Read the model definition and answer for the solid it produces. Units are mm, in the model's axes. A direction names the side the tool comes from. Give positions to 0.01 mm unless a question says otherwise; leave off trailing zeros. Write each loop counter-clockwise with the first axis right and the second up, starting at its lowest first coordinate (ties: lowest second). Pieces come first, ordered by that corner, then holes. Notation, with made-up numbers: (59.5, -30) - (89.5, -30) arc R25 ccw to (89.5, -15) - close; hole circle Ø6 at (36.5, -29). An arc over 180 degrees is marked (long way). Answer as a JSON object with one key per item and string values. Group by question number.
```python
from build123d import *

# Parameters (mm, degrees)
SKETCH1_W           = 40
SKETCH1_H           = 40
SKETCH1_R           = 2
SKETCH1_R_2         = 1.2
BOSS_EXTRUDE1_DEPTH = 4
SKETCH2_W           = 40
SKETCH2_H           = 40
BOSS_EXTRUDE2_DEPTH = 4
SKETCH3_W           = 7.5
SKETCH3_H           = 4
SKETCH3_W_2         = 20
SKETCH3_H_2         = 8
CUT_EXTRUDE1_DEPTH  = 4


with BuildPart() as part:
    # Sketch1 → Boss-Extrude1 (new body)
    with BuildSketch(Plane(origin=(0, 0, 0), x_dir=(1, 0, 0), z_dir=(0, 1, 0))):
        Rectangle(SKETCH1_W, SKETCH1_H)
        with Locations(Location((0, 0, 0), (0, 0, 270))):
            Circle(SKETCH1_R, mode=Mode.SUBTRACT)
        with Locations(Location((7, 0, 0), (0, 0, 270))):
            Circle(SKETCH1_R_2, mode=Mode.SUBTRACT)
        with Locations(Location((0, -7, 0), (0, 0, 270))):
            Circle(SKETCH1_R_2, mode=Mode.SUBTRACT)
        with Locations(Location((-7, 0, 0), (0, 0, 270))):
            Circle(SKETCH1_R_2, mode=Mode.SUBTRACT)
        with Locations(Location((0, 7, 0), (0, 0, 270))):
            Circle(SKETCH1_R_2, mode=Mode.SUBTRACT)
    extrude(amount=BOSS_EXTRUDE1_DEPTH)

    # Sketch2 → Boss-Extrude2 (add)
    with BuildSketch(Plane.XY.offset(20)):
        with Locations((0, 20)):
            Rectangle(SKETCH2_W, SKETCH2_H)
    extrude(amount=-BOSS_EXTRUDE2_DEPTH)

    # Sketch3 → Cut-Extrude1 (cut)
    with BuildSketch(Plane.XY.offset(20)):
        with Locations((-9.75, 30)):
            Rectangle(SKETCH3_W, SKETCH3_H)
        with Locations((9.75, 30)):
            Rectangle(SKETCH3_W, SKETCH3_H)
        with Locations((0, 12)):
            Rectangle(SKETCH3_W_2, SKETCH3_H_2)
    extrude(amount=-CUT_EXTRUDE1_DEPTH, mode=Mode.SUBTRACT)


solid = part.part
```
1) Find section D-D, the plane z = 7. Write down the section's boundary in (x, y), and give its area (3 significant figures).
2) Find the intervals of material crossed by line 1 (X direction, y = 1, z = 0); line 2 (X direction, y = 2, z = 7); line 3 (Z direction, x = 7.5, y = 25), in increasing order. Write a range as [from, to].
3) Find section C-C, the plane x = 0. Write down the section's boundary in (y, z).
4) Find section B-B, the plane x = -12.5. Write down the section's boundary in (y, z), and give its area (3 significant figures).
5) For a pull along Z with two mould halves and no side action, classify faces 4 (the cylindrical face through (0.05, 1.97, 5.8)), 5 (the flat face through (10, 12, 18)), 6 (the flat face through (0, 2, -20)) as released by +Z, released by -Z, zero draft, split by the parting line, or undercut.
6) Flat-ended cylindrical pins translate along their axes: pin 1 Ø3 at (x, z) = (0, 0) entering from -Y (3 decimals); pin 2 Ø4.5 at (x, z) = (8, 17.5) entering from -Y; pin 3 Ø1 at (x, z) = (-6, 2) entering from +Y; pin 4 Ø18 at (x, y) = (-3.5, 29) entering from -Z. Find the tip coordinate at first contact, or state that the pin passes through.
7) Find section A-A, the plane z = 0. Write down the section's boundary in (x, y), and give its area (3 significant figures).
8) Which of the six approach directions +Z, -Z, +X, -X, +Y, -Y give full straight-line access (tool end or side, diameter ignored) to faces 1 (the flat face through (10, 28, 18)), 2 (the flat face through (-0.3, 4, -2.3)), 3 (the flat face through (-20, 11, 16.4))?
Values follow:
{
 "1": {"outline": "(-20, 0) - (-1.2, 0) - (-1.2, 4) - (-20, 4) - close; (1.2, 0) - (20, 0) - (20, 4) - (1.2, 4) - close", "area": "150 mm2"},
 "2": {"line 1": "x = [-20, -8.2], [-5.8, -2], [2, 5.8], [8.2, 20]", "line 2": "x = [-20, -1.2], [1.2, 20]", "line 3": "z = [16, 20]"},
 "3": {"outline": "(0, -20) - (4, -20) - (4, -8.2) - (0, -8.2) - close; (0, -5.8) - (4, -5.8) - (4, -2) - (0, -2) - close; (0, 2) - (4, 2) - (4, 5.8) - (0, 5.8) - close; (0, 8.2) - (4, 8.2) - (4, 16) - (8, 16) - (8, 20) - (0, 20) - close; (16, 16) - (40, 16) - (40, 20) - (16, 20) - close"},
 "4": {"outline": "(0, -20) - (4, -20) - (4, 16) - (28, 16) - (28, 20) - (0, 20) - close; (32, 16) - (40, 16) - (40, 20) - (32, 20) - close", "area": "288 mm2"},
 "5": {"face 4": "undercut", "face 5": "zero draft", "face 6": "released by -Z"},
 "6": {"pin 1": "passes through", "pin 2": "stops at y = 0", "pin 3": "stops at y = 4", "pin 4": "stops at z = 16"},
 "7": {"outline": "(-20, 0) - (-8.2, 0) - (-8.2, 4) - (-20, 4) - close; (-5.8, 0) - (-2, 0) - (-2, 4) - (-5.8, 4) - close; (2, 0) - (5.8, 0) - (5.8, 4) - (2, 4) - close; (8.2, 0) - (20, 0) - (20, 4) - (8.2, 4) - close", "area": "125 mm2"},
 "8": {"face 1": "+Z, -Z", "face 2": "-Z, +X, -X, +Y", "face 3": "+Z, -Z, -X, +Y, -Y"}
}
